CAD build for the part. Positions are in the model's coordinates, mm. A direction names the side the tool comes from. Coordinates: 2 decimals unless noted, no trailing zeros. Order: outer loops, then holes, each group sorted by start corner. A loop starts at its lowest first (then second) coordinate and runs counter-clockwise, first axis right, second up. Notation, with made-up numbers: M 68.5,86.25 L 83.5,86.25 A15 cw 83.5,114.25 Z; hole C 83,70.25 d6. An arc over 180 degrees is marked long. Write item = value, one per line.
from build123d import *

# Parameters (mm, degrees)
SKETCH1_R           = 1.35255
BOSS_EXTRUDE1_DEPTH = 15.875
SKETCH2_R           = 4.7625
BOSS_EXTRUDE2_DEPTH = 1.5875
SKETCH3_R           = 3.3274
BOSS_EXTRUDE3_DEPTH = 1.8542
FILLET1_R           = 1.27
CUT_EXTRUDE1_DEPTH  = 1.8542


with BuildPart() as part:
    # Sketch1 → Boss-Extrude1 (new body)
    with BuildSketch(Plane.XY):
        Circle(SKETCH1_R)
    extrude(amount=BOSS_EXTRUDE1_DEPTH)

    # Sketch2 → Boss-Extrude2 (add)
    with BuildSketch(Plane.XY.offset(15.875)):
        Circle(SKETCH2_R)
    extrude(amount=BOSS_EXTRUDE2_DEPTH)

    # Sketch3 → Boss-Extrude3 (add)
    with BuildSketch(Plane.XY.offset(17.4625)):
        Circle(SKETCH3_R)
    extrude(amount=BOSS_EXTRUDE3_DEPTH)

    # Fillet1
    fillet1_edges = [part.edges().sort_by_distance(p)[0] for p in [
        (-3.3274, 0, 19.3167),
    ]]
    fillet(fillet1_edges, radius=FILLET1_R)

    # Sketch4 → Cut-Extrude1 (cut)
    with BuildSketch(Plane.XY.offset(19.3167)):
        Polygon((1.087800583, 0.359543143), (0.232526796, 1.121834511), (-0.855273787, 0.762291368), (-1.087800583, -0.359543143), (-0.232526796, -1.121834511), (0.855273787, -0.762291368), align=None)
    extrude(amount=-CUT_EXTRUDE1_DEPTH, mode=Mode.SUBTRACT)


solid = part.part
(1) Pin check, flat tips, straight feed: pin 1 Ø3 at (x, z) = (3.5, 2.5) entering from -Y; pin 2 Ø1.1 at (x, y) = (0, 0) entering from +Z; pin 3 Ø5 at (y, z) = (-2.5, 3.5) entering from +X; pin 4 Ø4 at (y, z) = (1, 13) entering from -X. Stop position of each tip, or through.
Evaluation:
pin_1 = through
pin_2 = 17.46
pin_3 = 1.35
pin_4 = -1.35
(2) Tool access for faces 5 (the face through (-1.1, 1.1, 15.875)), 6 (the face through (1, -1, 19.317)), 7 (the face through (-0.97, 0.21, 18.4)): list every direction of +Z, -Z, +X, -X, +Y, -Y with a clear straight run to the whole face (end or side of a thin tool).
Evaluation:
face_5 = -Z
face_6 = +Z, +X, -X, +Y, -Y
face_7 = +Z
(3) Pull direction X, two halves, no side cores. Call faces 1 (the face through (-3.78, -2.9, 16.66)), 2 (the face through (0, 0, 0)), 3 (the face through (0, 0, 17.463)), 4 (the face through (0.97, -0.21, 18.4)): +X half, -X half, draft (parallel to the pull), parting line (faces both ways), or undercut.
Evaluation:
face_1 = parting line
face_2 = draft
face_3 = undercut
face_4 = undercut
(4) Slice it at A-A, the plane z = 17.75. Write the cut outline in (x, y), then the cut area to 3 significant figures.
Evaluation:
outline = C 0,0 d6.65; hole M -1.09,-0.36 L -0.23,-1.12 L 0.86,-0.76 L 1.09,0.36 L 0.23,1.12 L -0.86,0.76 Z
area = 31.4 mm²
(5) Slice it at D-D, the plane z = 2.75. Write the cut outline in (x, y), then the cut area to 3 significant figures.
Evaluation:
outline = C 0,0 d2.71
area = 5.75 mm²
(6) Slice it at B-B, the plane x = 0. Write the cut outline in (y, z) (1 decimal), then the cut area to 3 significant figures.
Evaluation:
outline = M -4.8,15.9 L -1.4,15.9 L -1.4,0 L 1.4,0 L 1.4,15.9 L 4.8,15.9 L 4.8,17.5 L 3.3,17.5 L 3.3,18 A1.3 ccw 2.1,19.3 L 1,19.3 L 1,17.5 L -1,17.5 L -1,19.3 L -2.1,19.3 A1.3 ccw -3.3,18 L -3.3,17.5 L -4.8,17.5 Z
area = 65.8 mm²
(7) Wall check: line 1 (Z direction, x = -1.75, y = 1.25) (3 decimals); line 2 (Z direction, x = 0.75, y = -3.75) (1 decimal); line 3 (X direction, y = 0.75, z = 4.25). Give the ranges that are in metal, low to high. Write a range as from..to.
Evaluation:
line_1 = 15.875..19.313
line_2 = 15.9..17.5
line_3 = -1.13..1.13
